Check sheet for the drawn part. Datum: minimum x, y, z corner. Units: mm. A direction names the side the tool comes from. Give positions to 0.01 mm unless a question says otherwise; leave off trailing zeros. Order: outer loops, then holes, each group sorted by start corner. A loop starts at its lowest first (then second) coordinate and runs counter-clockwise, first axis right, second up. Notation, with made-up numbers: (83.25, 24.5) -> (114.25, 24.5) arc R29 ccw to (114.25, 53.5) -> close; hole circle Ø3 at (9, 81.5). An arc over 180 degrees is marked (long way). Answer in a Markdown table with one row per item. Add a question column.
(1) Cross-section at B-B (y = 27). Record the cut outline in (x, z).
(2) Cross-section at C-C (x = 88). Record the cut outline in (y, z).
(3) Cross-section at A-A (y = 6.5). Record the cut outline in (x, z).
(4) Thickness scan on L1, parallel to X at y = 14.5, z = 1.9; L2, parallel to Y at x = 19.5, z = 0.7; L3, parallel to Y at x = 103, z = 1.5. Record the ranges inside material, lowest first. Write a range as [from, to].
(5) Cross-section at D-D (y = 21). Record the cut outline in (x, z), then the cut area to 3 significant figures.
(6) Go/stop test with flat-tipped pins: pin 1 (3 mm diameter, centred on y = 13.5, z = 3, fed in from -X); pin 2 (2.5 mm diameter, centred on y = 10, z = 3, fed in from -X); pin 3 (1.2 mm diameter, centred on x = 78, z = 2, fed in from -Y); pin 4 (1.6 mm diameter, centred on x = 81.5, z = 3.5, fed in from -Y). Record where each tip stops, or that it passes through.
(7) Set-up check for the marked faces 4 and 5: record each of +Z, -Z, +X, -X, +Y, -Y from which the full face is reachable in a straight line by a thin tool's end or side.
(8) Release check for a two-part mould opening along Z. For the marked faces 1, 2 and 3 record: released by +Z, released by -Z, zero draft, split by the parting line, or undercut.
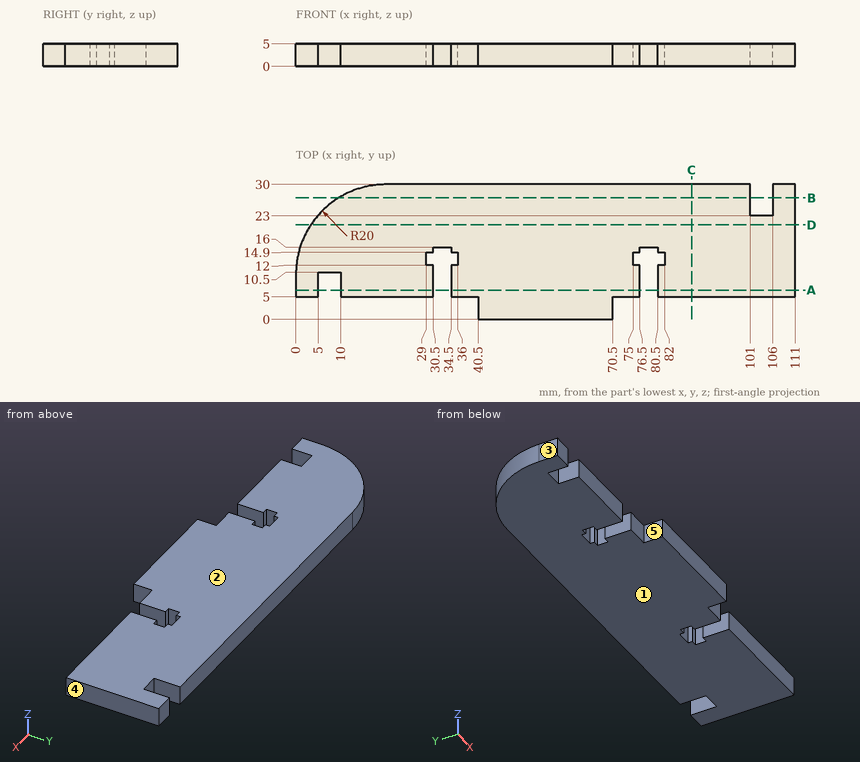
Answer below:
| question | item | result |
|---|---|---|
| 1 | outline | (9.46, 0) -> (101, 0) -> (101, 5) -> (9.46, 5) -> close; (106, 0) -> (111, 0) -> (111, 5) -> (106, 5) -> close |
| 2 | outline | (5, 0) -> (30, 0) -> (30, 5) -> (5, 5) -> close |
| 3 | outline | (0, 0) -> (5, 0) -> (5, 5) -> (0, 5) -> close; (10, 0) -> (30.5, 0) -> (30.5, 5) -> (10, 5) -> close; (34.5, 0) -> (76.5, 0) -> (76.5, 5) -> (34.5, 5) -> close; (80.5, 0) -> (111, 0) -> (111, 5) -> (80.5, 5) -> close |
| 4 | L1 | x = [0.51, 29], [36, 75], [82, 111] |
| 4 | L2 | y = [5, 29.99] |
| 4 | L3 | y = [5, 23] |
| 5 | outline | (3.3, 0) -> (111, 0) -> (111, 5) -> (3.3, 5) -> close |
| 5 | area | 539 mm² |
| 6 | pin 1 | stops at x = 0.1 |
| 6 | pin 2 | stops at x = 0 |
| 6 | pin 3 | stops at y = 16 |
| 6 | pin 4 | stops at y = 5 |
| 7 | face 4 | +Z, -Z, +X, +Y, -Y |
| 7 | face 5 | +Z, -Z, -X, -Y |
| 8 | face 1 | released by -Z |
| 8 | face 2 | released by +Z |
| 8 | face 3 | zero draft |
